Could you check a few things on this model? Use its own coordinates, in mm. Give positions to 0.01 mm unless a question says otherwise; leave off trailing zeros. Loops run counter-clockwise (first coordinate to the right, second up) from the corner with the lowest first, then second, coordinate; pieces in that order, holes last. Notation, with made-up numbers: (33.5, -2) - (51.5, -2) arc R32 cw to (51.5, 33) - close; hole circle Ø5 at (-6.75, 10). An arc over 180 degrees is marked (long way). Write each question's results on one line, items separated by ' | '. Start each with the question number.
1) I want a section at B-B, the plane x = 0. Write out the boundary of the cut face in (y, z), and give its area (3 significant figures).
2) I'm going to push flat-ended pins straight in: pin 1 (2 mm diameter, centred on x = -7, z = 2.5, fed in from -Y); pin 2 (5 mm diameter, centred on x = -11.67, y = 11.67, fed in from -Z); pin 3 (2 mm diameter, centred on x = 11, z = 5, fed in from +Y). Where does each tip first touch, or does it pass through?
3) I want a section at C-C, the plane x = -16.5. Write out the boundary of the cut face in (y, z), and give its area (3 significant figures).
4) I want a section at A-A, the plane y = 0. Write out the boundary of the cut face in (x, z), and give its area (3 significant figures).
5) If we mould it in two halves opening along Y, with no side actions, what happens to faces 1 (the face through (10, 5, 6.35)), 2 (the face through (-0.26, -14.523, 3.131)), 3 (the face through (10.382, -19.961, 3.131))? For each: +Y half, -Y half, draft (parallel to the pull), parting line (faces both ways), or undercut.
6) If I drill on probe 1 along Y at (x, z) = (0, 1.75); probe 2 along X at (y, z) = (1.5, 1.25); probe 3 along Y at (x, z) = (-10, 5.5), over which ranges is the centre line in solid material (lowest first)? Write a range as [from, to].
from build123d import *

# Parameters (mm, degrees)
SKETCH1_R             = 22.5
SKETCH1_R_2           = 11
SKETCH1_R_3           = 1.9939
SKETCH1_R_4           = 1.89865
BOSS_EXTRUDE1_DEPTH   = 6.35
CHAMFER1_SIZE         = 2.301024407
CHAMFER1_SIZE2        = 2.00025
CHAMFER1_PART_2_SIZE  = 2.301024407
CHAMFER1_PART_2_SIZE2 = 2.00025
CHAMFER1_PART_3_SIZE  = 2.301024407
CHAMFER1_PART_3_SIZE2 = 2.00025


with BuildPart() as part:
    # Sketch1 → Boss-Extrude1 (new body)
    with BuildSketch(Plane.XY):
        Circle(SKETCH1_R)
        Circle(SKETCH1_R_2, mode=Mode.SUBTRACT)
        with Locations((0, 16.5)):
            Circle(SKETCH1_R_3, mode=Mode.SUBTRACT)
        with Locations((11.66726189, 11.66726189)):
            Circle(SKETCH1_R_4, mode=Mode.SUBTRACT)
        with Locations((0, -16.5)):
            Circle(SKETCH1_R_3, mode=Mode.SUBTRACT)
        with Locations((-11.66726189, -11.66726189)):
            Circle(SKETCH1_R_4, mode=Mode.SUBTRACT)
        with Locations((-16.5, 0)):
            Circle(SKETCH1_R_3, mode=Mode.SUBTRACT)
        with Locations((-11.66726189, 11.66726189)):
            Circle(SKETCH1_R_4, mode=Mode.SUBTRACT)
    extrude(amount=BOSS_EXTRUDE1_DEPTH)

    # Chamfer1
    chamfer1_edges = [part.edges().sort_by_distance(p)[0] for p in [
        (9.76861189, 11.66726189, 0),
    ]]
    chamfer1_side = [part.faces().sort_by_distance(p)[0] for p in [
        (9.76861189, 11.66726189, 3.175),
    ]]
    chamfer(chamfer1_edges, length=CHAMFER1_SIZE, length2=CHAMFER1_SIZE2, reference=chamfer1_side[0])

    # Chamfer1 part 2
    chamfer1_part_2_edges = [part.edges().sort_by_distance(p)[0] for p in [
        (-13.56591189, -11.66726189, 0),
    ]]
    chamfer1_part_2_side = [part.faces().sort_by_distance(p)[0] for p in [
        (-13.56591189, -11.66726189, 3.175),
    ]]
    chamfer(chamfer1_part_2_edges, length=CHAMFER1_PART_2_SIZE, length2=CHAMFER1_PART_2_SIZE2, reference=chamfer1_part_2_side[0])

    # Chamfer1 part 3
    chamfer1_part_3_edges = [part.edges().sort_by_distance(p)[0] for p in [
        (-13.56591189, 11.66726189, 0),
    ]]
    chamfer1_part_3_side = [part.faces().sort_by_distance(p)[0] for p in [
        (-13.56591189, 11.66726189, 3.175),
    ]]
    chamfer(chamfer1_part_3_edges, length=CHAMFER1_PART_3_SIZE, length2=CHAMFER1_PART_3_SIZE2, reference=chamfer1_part_3_side[0])


solid = part.part
Answers:
1) outline: (-22.5, 0) - (-18.49, 0) - (-18.49, 6.35) - (-22.5, 6.35) - close; (-14.51, 0) - (-11, 0) - (-11, 6.35) - (-14.51, 6.35) - close; (11, 0) - (14.51, 0) - (14.51, 6.35) - (11, 6.35) - close; (18.49, 0) - (22.5, 0) - (22.5, 6.35) - (18.49, 6.35) - close | area: 95.4 mm2
2) pin 1: stops at y = -21.69 | pin 2: stops at z = 1.6 | pin 3: stops at y = 20.16
3) outline: (-15.3, 0) - (-1.99, 0) - (-1.99, 6.35) - (-15.3, 6.35) - close; (1.99, 0) - (15.3, 0) - (15.3, 6.35) - (1.99, 6.35) - close | area: 169 mm2
4) outline: (-22.5, 0) - (-18.49, 0) - (-18.49, 6.35) - (-22.5, 6.35) - close; (-14.51, 0) - (-11, 0) - (-11, 6.35) - (-14.51, 6.35) - close; (11, 0) - (22.5, 0) - (22.5, 6.35) - (11, 6.35) - close | area: 121 mm2
5) face 1: draft | face 2: undercut | face 3: parting line
6) probe 1: y = [-22.5, -18.49], [-14.51, -11], [11, 14.51], [18.49, 22.5] | probe 2: x = [-22.45, -17.81], [-15.19, -10.9], [10.9, 22.45] | probe 3: y = [-20.16, -12.58], [-10.76, -4.58], [4.58, 10.76], [12.58, 20.16]
